CAD build for the part. Positions are in the model's coordinates, mm. A direction names the side the tool comes from. Round coordinates to 2 decimals unless told otherwise and drop trailing zeros. Order: outer loops, then holes, each group sorted by start corner. A loop starts at its lowest first (then second) coordinate and runs counter-clockwise, first axis right, second up. Notation, with made-up numbers: M 60,-20 L 65,-20 A11 cw 65,-6 Z; hole C 5,-27.75 d5. An arc over 180 degrees is marked long. Put each result on its own line as item: value.
```python
from build123d import *

# Parameters (mm, degrees)
ESQUISSE1_W        = 40
ESQUISSE1_H        = 40
BOSS_EXTRU_1_DEPTH = 56
ESQUISSE2_R        = 18
BOSS_EXTRU_2_DEPTH = 38
ESQUISSE3_R        = 11.5
BOSS_EXTRU_3_DEPTH = 2
ESQUISSE4_W        = 12.050195296
ESQUISSE4_H        = 4.136634206
BOSS_EXTRU_4_DEPTH = 16


with BuildPart() as part:
    # Esquisse1 → Boss.-Extru.1 (new body)
    with BuildSketch(Plane.XY):
        with Locations((20, 20)):
            Rectangle(ESQUISSE1_W, ESQUISSE1_H)
    extrude(amount=BOSS_EXTRU_1_DEPTH)

    # Esquisse2 → Boss.-Extru.2 (add)
    with BuildSketch(Plane.XY.offset(56)):
        with Locations((20, 20)):
            Circle(ESQUISSE2_R)
    extrude(amount=BOSS_EXTRU_2_DEPTH)

    # Esquisse3 → Boss.-Extru.3 (add)
    with BuildSketch(Plane.XY.offset(94)):
        with Locations((20, 20)):
            Circle(ESQUISSE3_R)
    extrude(amount=BOSS_EXTRU_3_DEPTH)

    # Esquisse4 → Boss.-Extru.4 (add)
    with BuildSketch(Plane.XY.offset(96)):
        with Locations((20, 20)):
            Rectangle(ESQUISSE4_W, ESQUISSE4_H)
    extrude(amount=BOSS_EXTRU_4_DEPTH)


solid = part.part
```
Item 1: Band-saw the part on D-D on x = 12.5. Give the cut face in (y, z).
Answers below:
outline: M 0,0 L 40,0 L 40,56 L 36.36,56 L 36.36,94 L 28.72,94 L 28.72,96 L 11.28,96 L 11.28,94 L 3.64,94 L 3.64,56 L 0,56 Z
Item 2: Band-saw the part on B-B on x = 20. Give the cut face in (y, z), and give its area (3 significant figures).
Answers below:
outline: M 0,0 L 40,0 L 40,56 L 38,56 L 38,94 L 31.5,94 L 31.5,96 L 22.07,96 L 22.07,112 L 17.93,112 L 17.93,96 L 8.5,96 L 8.5,94 L 2,94 L 2,56 L 0,56 Z
area: 3,720 mm²
Item 3: Band-saw the part on C-C on z = 88.5. Give the cut face in (x, y).
Answers below:
outline: C 20,20 d36
Item 4: Pin check, flat tips, straight feed: P1, Ø13.5, axis at x = 18, z = 105, coming from the -Y side; P2, Ø13.5, axis at x = 18, z = 103.5, coming from the +Y side; P3, Ø1, axis at y = 34.5, z = 87, coming from the +X side. Stop position of each tip, or through.
Answers below:
P1: y = 17.93
P2: y = 22.07
P3: x = 31.31
Item 5: Tool access for faces 1 (the flat face through (15, 38, 56)), 2 (the flat face through (20, 22.068, 104)), 3 (the flat face through (20, 17.932, 104)), 4 (the flat face through (13.975, 20, 104)): list every direction of +Z, -Z, +X, -X, +Y, -Y with a clear straight run to the whole face (end or side of a thin tool).
Answers below:
face 1: +Z
face 2: +Z, +X, -X, +Y
face 3: +Z, +X, -X, -Y
face 4: +Z, -X, +Y, -Y
Item 6: Probe line 1 along Z through (x, y) = (3, 36); line 2 along Z through (x, y) = (17.5, 33); line 3 along Y through (x, z) = (25, 107.5). List the from-to ranges inside material, lowest first. Write a range as [from, to].
Answers below:
line 1: [0, 56]
line 2: [0, 94]
line 3: [17.93, 22.07]
Item 7: Band-saw the part on A-A on y = 20. Give the cut face in (x, z).
Answers below:
outline: M 0,0 L 40,0 L 40,56 L 38,56 L 38,94 L 31.5,94 L 31.5,96 L 26.03,96 L 26.03,112 L 13.97,112 L 13.97,96 L 8.5,96 L 8.5,94 L 2,94 L 2,56 L 0,56 Z
